```python
from build123d import *

# Parameters (mm, degrees)
SKETCH1_R           = 4
BOSS_EXTRUDE1_DEPTH = 10
BOSS_EXTRUDE2_DEPTH = 3
SKETCH3_R           = 4.5
SKETCH3_R_2         = 4
BOSS_EXTRUDE3_DEPTH = 3


with BuildPart() as part:
    # Sketch1 → Boss-Extrude1 (new body)
    with BuildSketch(Plane(origin=(0, 0, 0), x_dir=(1, 0, 0), z_dir=(0, 1, 0))):
        with Locations(Location((0, 0, 0), (0, 0, 270))):
            Circle(SKETCH1_R)
    extrude(amount=BOSS_EXTRUDE1_DEPTH)

    # Sketch2 → Boss-Extrude2 (add)
    with BuildSketch(Plane(origin=(0, 10, 0), x_dir=(1, 0, 0), z_dir=(0, 1, 0))):
        with BuildLine():
            Line((1.457625029, 1.5), (-1.457625029, 1.5))
            ThreePointArc((-1.457625029, 1.5), (-0.814230917, -1.926576949), (2.091571353, 0))
            ThreePointArc((2.091571353, 0), (1.926576949, 0.814230917), (1.457625029, 1.5))
        make_face()
    extrude(amount=BOSS_EXTRUDE2_DEPTH)

    # Sketch3 → Boss-Extrude3 (add)
    with BuildSketch(Plane.XZ):
        with Locations(Location((0, 0, 0), (0, 0, 270))):
            Circle(SKETCH3_R)
        with Locations(Location((0, 0, 0), (0, 0, 270))):
            Circle(SKETCH3_R_2, mode=Mode.SUBTRACT)
    extrude(amount=-BOSS_EXTRUDE3_DEPTH)


solid = part.part
```
Source: CAD feature listing. Evaluate the final solid. Frame: model axes, mm. A direction names the side the tool comes from. Round coordinates to 2 decimals unless told otherwise and drop trailing zeros. Loops run counter-clockwise (first coordinate to the right, second up) from the corner with the lowest first, then second, coordinate; pieces in that order, holes last. Notation, with made-up numbers: M 45.5,-9.75 L 49.5,-9.75 A3 ccw 49.5,-5.75 Z; hole C 43.25,-14.75 d4. An arc over 180 degrees is marked long. Use a Markdown table: item, result. Add a question column.
1. Contact query for flat-ended pins moving along their axis: P1, Ø4, axis at x = 2.5, y = 4, coming from the -Z side; P2, Ø3, axis at x = 0, y = 6, coming from the +Z side; P3, Ø0.9, axis at x = 0.5, y = 12, coming from the -Z side; P4, Ø3, axis at y = 2.5, z = 1.5, coming from the -X side. Output: stop coordinate, or through.
2. Section query A-A on x = 0. Return the cut outline in (y, z).
3. Section query C-C on y = 3.75. Return the cut outline in (x, z), then the cut area to 3 significant figures.
4. Reachability of faces 1 (the cylindrical face through (-3.905, 6.451, -0.867)), 2 (the flat face through (0, 11, -1.5)), 3 (the flat face through (0, 13, 0)) from +Z, -Z, +X, -X, +Y, -Y: full face, straight path, thin tool, end or side. Return the list, or none.
5. Section query D-D on x = -2.5. Return the cut outline in (y, z).
6. Line query: line 1 (Y direction, x = -0.25, z = 2.5); line 2 (Z direction, x = -1.5, y = 12); line 3 (Y direction, x = -3.5, z = 2.5). Output: solid intervals per line, ascending.
7. Section query B-B on z = 2.25. Return the cut outline in (x, y).
Reported:
| question | item | result |
|---|---|---|
| 1 | P1 | stops at z = -4.43 |
| 1 | P2 | stops at z = 4 |
| 1 | P3 | stops at z = -1.5 |
| 1 | P4 | stops at x = -4.5 |
| 2 | outline | M 0,-4.5 L 3,-4.5 L 3,-4 L 10,-4 L 10,-1.5 L 13,-1.5 L 13,2.09 L 10,2.09 L 10,4 L 3,4 L 3,4.5 L 0,4.5 Z |
| 3 | outline | C 0,0 d8 |
| 3 | area | 50.3 mm² |
| 4 | face 1 | +Y |
| 4 | face 2 | -Z, +X, -X, +Y |
| 4 | face 3 | +Z, -Z, +X, -X, +Y |
| 5 | outline | M 0,-3.74 L 3,-3.74 L 3,-3.12 L 10,-3.12 L 10,3.12 L 3,3.12 L 3,3.74 L 0,3.74 Z |
| 6 | line 1 | y = 0 to 10 |
| 6 | line 2 | z = -1.46 to 1.46 |
| 6 | line 3 | y = 0 to 3 |
| 7 | outline | M -3.9,0 L 3.9,0 L 3.9,3 L 3.31,3 L 3.31,10 L -3.31,10 L -3.31,3 L -3.9,3 Z |
